For this review, take the finished solid that the model builds, in its own axes (mm). A direction names the side the tool comes from. Give positions to 0.01 mm unless a question says otherwise; leave off trailing zeros. Order: outer loops, then holes, each group sorted by start corner. A loop starts at its lowest first (then second) coordinate and runs counter-clockwise, first axis right, second up. Notation, with made-up numbers: (41.25, 48.5) -> (69.25, 48.5) arc R27 ccw to (69.25, 83.5) -> close; hole circle Ø6 at (78.25, 64). An arc over 180 degrees is marked (long way). Return JSON: item names as keys, results as strings. Group by question number.
1) Insertion check: P1, Ø3.5, axis at x = 0, y = 80, coming from the -Z side; P2, Ø1, axis at y = 83, z = 1, coming from the -X side; P3, Ø2.5, axis at x = -2, y = 78, coming from the +Z side; P4, Ø1, axis at x = 4.5, y = 86.5, coming from the +Z side. Each pin has a flat end and moves straight along its axis. Give the tip position at first contact, or say it passes through.
2) The part is to be moulded in two halves that separate along X. For faces 4 (the face through (-13.5, 67, 6)), 5 (the face through (2, 18, 1)), 6 (the face through (-9, 67, 1.5)), say which applies: released by +X, released by -X, zero draft, split by the parting line, or undercut.
3) To check wall thickness, follow line 1 along Y through (x, z) = (0, 0.4); line 2 along Y through (x, z) = (0, 2.6); line 3 along X through (y, z) = (76, 6). State the ranges of each line that lie inside material, in increasing order.
4) Add section A-A (x = 0). Give the boundary of the cut face in (y, z), then the cut area to 3 significant figures.
5) For faces 1 (the face through (-10, 67, 3)), 2 (the face through (1.96, 76.23, 2.57)), 3 (the face through (10, 69, 7.6)), list the 3-axis set-ups (+Z, -Z, +X, -X, +Y, -Y) from which the entire face can be reached by the end or side of a thin tool; tool diameter is ignored.
from build123d import *

# Parameters (mm, degrees)
BOSS_EXTRU_1_DEPTH                                 = 1000
ENL_V_MAT_EXTRU_1_DEPTH                            = 1001
CHAMBRAGE_POUR_VIS_T_TE_HEXAGONALE_M41_D           = 4.5
CHAMBRAGE_POUR_VIS_T_TE_HEXAGONALE_M41_DEPTH       = 4.1
CHAMBRAGE_POUR_VIS_T_TE_HEXAGONALE_M41_CBORE_D     = 8.5
CHAMBRAGE_POUR_VIS_T_TE_HEXAGONALE_M41_CBORE_DEPTH = 3.1
DIAM_TRE_DU_PER_AGE_0_4_0_4_1_D                    = 0.4
DIAM_TRE_DU_PER_AGE_0_4_0_4_1_DEPTH                = 1000
CONG_1_R                                           = 0.2
CONG_2_R                                           = 0.5
CONG_3_R                                           = 1
ESQUISSE9_W                                        = 27
ESQUISSE9_H                                        = 864.38
ENL_V_MAT_EXTRU_2_DEPTH                            = 9.7
ENL_V_MAT_EXTRU_2_DEPTH_BACK                       = 1


with BuildPart() as part:
    # Esquisse1 → Boss.-Extru.1 (new body)
    with BuildSketch(Plane.XZ):
        with BuildLine():
            Line((13.5, 8.7), (-13.5, 8.7))
            Line((-13.5, 8.7), (-13.5, 3))
            Line((-13.5, 3), (-7.8, 3))
            ThreePointArc((-7.8, 3), (-7.05, 2.25), (-7.8, 1.5))
            Line((-7.8, 1.5), (-11, 1.5))
            Line((-11, 1.5), (-11, 0))
            Line((-11, 0), (11, 0))
            Line((11, 0), (11, 1.5))
            Line((11, 1.5), (7.8, 1.5))
            ThreePointArc((7.8, 1.5), (7.05, 2.25), (7.8, 3))
            Line((7.8, 3), (13.5, 3))
            Line((13.5, 3), (13.5, 8.7))
        make_face()
    extrude(amount=-BOSS_EXTRU_1_DEPTH)

    # Esquisse2 → Enlèv. mat.-Extru.1 (cut, through all)
    with BuildSketch(Plane(origin=(0, 1000, 0), x_dir=(-1, 0, 0), z_dir=(0, 1, 0))):
        Polygon((8.75, 8.7), (-8.75, 8.7), (-8.75, 7.6), (-12, 7.6), (-12, 4.1), (12, 4.1), (12, 7.6), (8.75, 7.6), align=None)
    extrude(amount=-ENL_V_MAT_EXTRU_1_DEPTH, mode=Mode.SUBTRACT)

    # Chambrage pour vis à tête hexagonale M41
    with Locations(Plane.XY.offset(4.1)):
        with Locations((0, 980), (0, 920), (0, 860), (0, 800), (0, 740), (0, 680), (0, 620), (0, 560), (0, 500), (0, 440), (0, 380), (0, 320), (0, 260), (0, 200), (0, 140), (0, 80), (0, 20)):
            CounterBoreHole(CHAMBRAGE_POUR_VIS_T_TE_HEXAGONALE_M41_D / 2, CHAMBRAGE_POUR_VIS_T_TE_HEXAGONALE_M41_CBORE_D / 2, CHAMBRAGE_POUR_VIS_T_TE_HEXAGONALE_M41_CBORE_DEPTH, depth=CHAMBRAGE_POUR_VIS_T_TE_HEXAGONALE_M41_DEPTH)

    # Diamètre du perçage Ø0.4 (0.4)1
    with Locations(Plane(origin=(0, 0, 0), x_dir=(-1, 0, 0), z_dir=(0, -1, 0))):
        with Locations((7.75, -4.1), (-7.75, -4.1)):
            Hole(DIAM_TRE_DU_PER_AGE_0_4_0_4_1_D / 2, depth=DIAM_TRE_DU_PER_AGE_0_4_0_4_1_DEPTH)

    # Congé1
    cong_1_edges = [part.edges().sort_by_distance(p)[0] for p in [
        (11, 500, 1.5),
        (-11, 500, 1.5),
    ]]
    fillet(cong_1_edges, radius=CONG_1_R)

    # Congé2
    cong_2_edges = [part.edges().sort_by_distance(p)[0] for p in [
        (-12, 500, 7.6),
        (-12, 500, 4.1),
        (12, 500, 4.1),
        (12, 500, 7.6),
    ]]
    fillet(cong_2_edges, radius=CONG_2_R)

    # Congé3
    cong_3_edges = [part.edges().sort_by_distance(p)[0] for p in [
        (13.5, 500, 3),
        (-13.5, 500, 3),
        (-13.5, 500, 8.7),
        (13.5, 500, 8.7),
    ]]
    fillet(cong_3_edges, radius=CONG_3_R)

    # Esquisse9 → Enlèv. mat.-Extru.2 (cut, two sides)
    with BuildSketch(Plane.XY) as enl_v_mat_extru_2_sk:
        with Locations((0, 567.81)):
            Rectangle(ESQUISSE9_W, ESQUISSE9_H)
    extrude(amount=ENL_V_MAT_EXTRU_2_DEPTH, mode=Mode.SUBTRACT)
    extrude(enl_v_mat_extru_2_sk.sketch, amount=-ENL_V_MAT_EXTRU_2_DEPTH_BACK, mode=Mode.SUBTRACT)


solid = part.part
Evaluation:
{
 "1": {"P1": "through", "P2": "x = -11", "P3": "z = 1", "P4": "z = 4.1"},
 "2": {"face 4": "released by -X", "face 5": "undercut", "face 6": "zero draft"},
 "3": {"line 1": "0 to 17.75, 22.25 to 77.75, 82.25 to 135.62", "line 2": "0 to 15.75, 24.25 to 75.75, 84.25 to 135.62", "line 3": "-13.5 to -12, 12 to 13.5"},
 "4": {"outline": "(0, 0) -> (17.75, 0) -> (17.75, 1) -> (15.75, 1) -> (15.75, 4.1) -> (0, 4.1) -> close; (22.25, 0) -> (77.75, 0) -> (77.75, 1) -> (75.75, 1) -> (75.75, 4.1) -> (24.25, 4.1) -> (24.25, 1) -> (22.25, 1) -> close; (82.25, 0) -> (135.62, 0) -> (135.62, 4.1) -> (84.25, 4.1) -> (84.25, 1) -> (82.25, 1) -> close", "area": "494 mm^2"},
 "5": {"face 1": "-X, +Y, -Y", "face 2": "+Z", "face 3": "+Y, -Y"}
}
